from build123d import *

# Parameters (mm, degrees)
SKETCH_1_W          = 15
SKETCH_1_H          = 15
SKETCH_1_W_2        = 12
SKETCH_1_H_2        = 12
EXTRUDE_2_DEPTH     = 45
SKETCH_2_R          = 1.5
CUT_EXTRUDE_1_DEPTH = 10
SKETCH_3_R          = 1.5
CUT_EXTRUDE_2_DEPTH = 10
SKETCH_4_R          = 4
CUT_EXTRUDE_3_DEPTH = 10
SKETCH_5_R          = 4
CUT_EXTRUDE_4_DEPTH = 10


with BuildPart() as part:
    # ｽｹｯﾁ1 → ﾎﾞｽ - 押し出し2 (new body)
    with BuildSketch(Plane.XY):
        with Locations((0.489915859, 0.232626086)):
            Rectangle(SKETCH_1_W, SKETCH_1_H)
        with Locations((0.489915859, 0.232626086)):
            Rectangle(SKETCH_1_W_2, SKETCH_1_H_2, mode=Mode.SUBTRACT)
    extrude(amount=EXTRUDE_2_DEPTH)

    # ｽｹｯﾁ2 → ｶｯﾄ - 押し出し1 (cut)
    with BuildSketch(Plane(origin=(7.989915859, 0, 0), x_dir=(0, 0, -1), z_dir=(1, 0, 0))):
        with Locations((-22.5, 0.232626086)):
            Circle(SKETCH_2_R)
    extrude(amount=-CUT_EXTRUDE_1_DEPTH, mode=Mode.SUBTRACT)

    # ｽｹｯﾁ3 → ｶｯﾄ - 押し出し2 (cut)
    with BuildSketch(Plane.XZ.offset(7.267373914)):
        with Locations((0.489915859, 37.5)):
            Circle(SKETCH_3_R)
        with Locations((0.489915859, 7.5)):
            Circle(SKETCH_3_R)
    extrude(amount=-CUT_EXTRUDE_2_DEPTH, mode=Mode.SUBTRACT)

    # ｽｹｯﾁ4 → ｶｯﾄ - 押し出し3 (cut)
    with BuildSketch(Plane.ZY.offset(7.010084141)):
        with Locations((22.5, 0.232626086)):
            Circle(SKETCH_4_R)
    extrude(amount=-CUT_EXTRUDE_3_DEPTH, mode=Mode.SUBTRACT)

    # ｽｹｯﾁ5 → ｶｯﾄ - 押し出し4 (cut)
    with BuildSketch(Plane(origin=(0, 7.732626086, 0), x_dir=(1, 0, 0), z_dir=(0, 1, 0))):
        with Locations((0.489915859, -7.5)):
            Circle(SKETCH_5_R)
        with Locations((0.489915859, -37.5)):
            Circle(SKETCH_5_R)
    extrude(amount=-CUT_EXTRUDE_4_DEPTH, mode=Mode.SUBTRACT)


solid = part.part
Read the model definition and answer for the solid it produces. Units are mm, in the model's axes. A direction names the side the tool comes from. Round coordinates to 2 decimals unless told otherwise and drop trailing zeros. Loops run counter-clockwise (first coordinate to the right, second up) from the corner with the lowest first, then second, coordinate; pieces in that order, holes last. Notation, with made-up numbers: (15.25, 51.5) - (34.25, 51.5) arc R16 cw to (34.25, 71.5) - close; hole circle Ø6 at (21.25, -24.5). An arc over 180 degrees is marked (long way). One line per question, with ' | ' between items. Start each with the question number.
Q1. Section A-A on z = 15.5 is taken. Give the vertices of the cut face in (x, y), plus the area to 3 significant figures.
Q2. Section B-B on x = 6 is taken. Give the vertices of the cut face in (y, z).
Q3. For faces 5 (the flat face through (-5.51, -4, 22)), 6 (the cylindrical face through (-2.684, 6.993, 9.934)), 7 (the cylindrical face through (-6.271, 0.408, 18.504)), determine the directions among +Z, -Z, +X, -X, +Y, -Y from which every point of the face is accessible in a straight line to the end or side of a thin tool.
Q4. Flat-ended cylindrical pins translate along their axes: pin 1 (3.5 mm diameter, centred on x = 0.49, z = 37.5, fed in from +Y); pin 2 (6.5 mm diameter, centred on y = 0.23, z = 22.5, fed in from -X). Find the tip coordinate at first contact, or state that the pin passes through.
Q5. Section D-D on z = 22.5 is taken. Give the vertices of the cut face in (x, y), plus the area to 3 significant figures.
Q6. For a pull along Z with two mould halves and no side action, classify faces 1 (the flat face through (-6, 0, 45)), 2 (the cylindrical face through (0.165, -6.528, 6.036)), 3 (the flat face through (6.49, 3, 22)), 4 (the flat face through (-6, 0, 0)) as +Z half, -Z half, draft (parallel to the pull), parting line (faces both ways), or undercut.
Q7. Section C-C on y = -5 is taken. Give the vertices of the cut face in (x, z).
Q8. Find the intervals of material crossed by L1, parallel to X at y = -4.25, z = 13.5; L2, parallel to Z at x = -5.75, y = 0; L3, parallel to Y at x = -1.5, z = 26, in increasing order.
Established:
1) outline: (-7.01, -7.27) - (7.99, -7.27) - (7.99, 7.73) - (-7.01, 7.73) - close; hole (-5.51, -5.77) - (6.49, -5.77) - (6.49, 6.23) - (-5.51, 6.23) - close | area: 81.0 mm²
2) outline: (-7.27, 0) - (-5.77, 0) - (-5.77, 45) - (-7.27, 45) - close; (6.23, 0) - (7.73, 0) - (7.73, 45) - (6.23, 45) - close
3) face 5: +Z, -Z | face 6: +Y | face 7: -X
4) pin 1: y = -5.77 | pin 2: x = 6.49
5) outline: (-7.01, -7.27) - (7.99, -7.27) - (7.99, -1.27) - (6.49, -1.27) - (6.49, -5.77) - (-5.51, -5.77) - (-5.51, -3.77) - (-7.01, -3.77) - close; (-7.01, 4.23) - (-5.51, 4.23) - (-5.51, 6.23) - (6.49, 6.23) - (6.49, 1.73) - (7.99, 1.73) - (7.99, 7.73) - (-7.01, 7.73) - close | area: 64.5 mm²
6) face 1: +Z half | face 2: undercut | face 3: draft | face 4: -Z half
7) outline: (-7.01, 0) - (-5.51, 0) - (-5.51, 45) - (-7.01, 45) - close; (6.49, 0) - (7.99, 0) - (7.99, 45) - (6.49, 45) - close
8) L1: -7.01 to -5.51, 6.49 to 7.99 | L2: 0 to 18.51, 26.49 to 45 | L3: -7.27 to -5.77, 6.23 to 7.73
